Work out the finished part from the listing and answer in its coordinate system (mm). A direction names the side the tool comes from. Give positions to 0.01 mm unless a question says otherwise; leave off trailing zeros. Write each loop counter-clockwise with the first axis right and the second up, starting at its lowest first coordinate (ties: lowest second). Pieces come first, ordered by that corner, then holes.
1) Find section A-A (y = 0). Determine the outline of the cut face in (x, z), plus the area to 3 significant figures.
2) A tool of negligible diameter and unlimited length cuts with its end or side. For faces 1 (the face through (-5, 6, 12)), 2 (the face through (0, 4.8, -5.6)), 3 (the face through (0, -6, 12)), from which of +Z, -Z, +X, -X, +Y, -Y can it reach the whole face along a straight path? Write none if from no direction.
3) Straight lines are drawn through the part: probe 1 along X at (y, z) = (-4.25, -4.5); probe 2 along Y at (x, z) = (0, 3). For each, find the intervals that lie inside material, in ascending order.
4) Find section C-C (x = 0). Count the separate pieces of the cut face and the enclosed holes in it, plus the area to 3 significant figures.
5) Determine the mould class of faces 4 (the face through (0, -3, -15)), 5 (the face through (0, -4.8, -5.6)), 6 (the face through (-0.12, 4.02, -8.11)), 7 (the face through (-1.55, -5, 4)) for opening direction Z: pulls with the +Z half, pulls with the -Z half, needs draft (parallel to the pull), parting line crosses it, or undercut.
6) Given pin 1 Ø1.6 at (x, z) = (0, -9) entering from -Y; pin 2 Ø2 at (x, z) = (-5, 10.5) entering from +Y; pin 3 Ø5 at (x, z) = (-4.5, 4) entering from -Y; pin 4 Ø1.1 at (x, y) = (-2, -6.5) entering from +Z, each flat-ended and moving along its own axis, determine where each tip first touches the part or whether it passes through.
Autodesk Inventor part; units mm, degrees
ref_plane "Work Plane3" through (0, -6, 0) normal (0, 1, 0) x (-1, 0, 0)
ref_plane "YZ Plane" through (0, 0, 0) normal (1, 0, 0) x (0, 1, 0)
ref_plane "XY Plane" through (0, 0, 0) normal (0, 0, 1) x (1, 0, 0)
sketch "Sketch1" plane through (0, 0, 0) normal (0, 0, 1) x (1, 0, 0)
  line L0 (-2.1, -2.1) -> (2.1, -2.1)
  line L1 (2.1, -2.1) -> (2.1, 2.1)
  line L2 (2.1, 2.1) -> (-2.1, 2.1)
  line L3 (-2.1, 2.1) -> (-2.1, -2.1)
  line L4 (-2.1, -2.1) -> (2.1, 2.1) construction
  line L5 (2.1, -2.1) -> (-2.1, 2.1) construction
  line L6 (-6, -6) -> (6, -6)
  line L7 (6, -6) -> (6, 6)
  line L8 (6, 6) -> (-6, 6)
  line L9 (-6, 6) -> (-6, -6)
  line L10 (-6, -6) -> (6, 6) construction
  line L11 (6, -6) -> (-6, 6) construction
  line L12 (0, 6) -> (0, 2.1)
  point P0 (0, 0)
  dimension "d0" = 4.2
  dimension "d1" = 4.2
  dimension "d2" = 12
  dimension "d3" = 12
  dimension "d93" = 3.9
extrude "Extrusion1" add sketch "Sketch1" along normal mid plane 30
sketch "Sketch2" plane through (-6, 6, 15) normal (0, 1, 0) x (1, 0, 0)
  line L0 (0, 30) -> (0, 0)
  line L1 (0, 0) -> (0, 6)
  line L2 (0, 0) -> (0, 8)
  line L3 (0, 6) -> (12, 6)
  line L4 (12, 30) -> (12, 0)
  line L5 (0, 8) -> (12, 8)
  line L6 (12, 6) -> (12, 8)
  point P0 (6, 15)
  dimension "d6" = 6
  dimension "d7" = 8
  dimension "d8" = 2
extrude "Extrusion2" add sketch "Sketch2" along normal blind 2
sketch "Sketch3" plane through (-6, 6, -15) normal (0, 1, 0) x (1, 0, 0)
  line L0 (0, 0) -> (0, -30)
  line L1 (12, -30) -> (12, 0)
  line L2 (0, 0) -> (0, -22)
  line L3 (12, -30) -> (0, -30)
  line L4 (9.1, -31) -> (2.9, -31)
  line L5 (6, -6) -> (6, 0)
  circle A0 centre (6, -6) radius 1.55
  line L6 (2.8, -31) -> (4, -31)
  line L7 (9.2, -31) -> (8, -31)
  circle A1 centre (6, -6) radius 3.4
  line L8 (2.6, -6) -> (2.6, -31)
  line L9 (2.6, -6) -> (27.6, -6) construction
  line L10 (2.6, -31) -> (4, -31)
  line L11 (9.4, -6) -> (9.4, -31)
  line L12 (9.4, -6) -> (34.4, -6) construction
  line L13 (9.4, -31) -> (8, -31)
  line L14 (4.45, -6) -> (4.45, -31)
  line L15 (4.45, -6) -> (29.45, -6) construction
  line L16 (7.55, -6) -> (7.55, -31)
  line L17 (7.55, -6) -> (32.55, -6) construction
  point P0 (6, -15)
  point P1 (9.4, -30)
  point P2 (2.6, -30)
  point P3 (4.45, -30)
  point P4 (4.45, -9.0261)
  point P5 (7.55, -9.0261)
  point P6 (7.55, -30)
  dimension "d139" = 6
  dimension "d145" = 3.1
  dimension "d183" = 6.8
  dimension "d184" = 90
  dimension "d185" = 90
  dimension "d190" = 90
  dimension "d191" = 90
  dimension "d204" = 6
extrude "Extrusion3" cut sketch "Sketch3" against normal blind 2.5 contours L3 L16 A1 L11 | A1 L16 A0 L5 | L3 L8 A1 L14 | A1 L14 A0 L16 | L5 A0 L14 A1
ref_plane "Work Plane3" through (0, -6, 0) normal (0, 1, 0) x (-1, 0, 0)
sketch "Sketch16" plane through (-6, -6, -15) normal (0, -1, 0) x (1, 0, 0)
  line L0 (12, 0) -> (0, 0)
  line L1 (0, 0) -> (6, 0)
  line L2 (6, 0) -> (6, 6)
  circle A0 centre (6, 6) radius 1.55
  arc A1 (7.55, 6) -> (7.55, 6) centre (6, 6) ccw
  line L3 (10.2, 6) -> (36.7126, 6) construction
  line L4 (8.95, 32.5126) -> (7.75, 32.5126)
  line L5 (2.8, 6) -> (29.3126, 6) construction
  line L6 (7.55, 6) -> (9.4, 6)
  circle A2 centre (6, 6) radius 3.4
  line L7 (9.4, 6) -> (9.4, 32.5126)
  line L8 (9.4, 6) -> (35.9126, 6) construction
  line L9 (9.4, 32.5126) -> (7.75, 32.5126)
  line L10 (2.6, 6) -> (2.6, 32.5126)
  line L11 (2.6, 6) -> (29.1126, 6) construction
  line L12 (7.55, 6) -> (7.55, 32.5126)
  line L13 (7.55, 6) -> (34.0626, 6) construction
  line L14 (7.55, 32.5126) -> (9.4, 32.5126)
  line L15 (4.45, 6) -> (4.45, 32.5126)
  line L16 (4.45, 6) -> (30.9626, 6) construction
  line L17 (4.45, 32.5126) -> (2.6, 32.5126)
  point P0 (10.1, 6)
  point P1 (4.45, 9.0261)
  point P2 (7.55, 9.0261)
  dimension "d155" = 6
  dimension "d156" = 6
  dimension "d181" = 90
  dimension "d182" = 90
  dimension "d187" = 3.1
  dimension "d188" = 90
  dimension "d189" = 90
  dimension "d198" = 6.8
extrude "Extrusion12" cut sketch "Sketch16" against normal blind 2.5 contours A2 L15 A0 L2 | L2 A0 L6 A2 | L10 L17 L15 A2 | L6 L12 A2 | A2 L12 L14 L4 L9 L7 | L15 A2 L12 A0
sketch "Sketch17" plane through (0, -6, -9) normal (0, -1, 0) x (1, 0, 0)
  circle A0 centre (0, 0) radius 0.9
  point P0 (0, 9)
  point P1 (3.1, 0)
  dimension "d186" = 1.8
extrude "Extrusion13" cut sketch "Sketch17" against normal through all
sketch "Sketch18" plane through (0, -6, -9) normal (0, -1, 0) x (1, 0, 0)
  line L0 (0, 0) -> (0, 1)
  arc A0 (-7, 1) -> (7, 1) centre (0, 1) ccw
  line L1 (0, 1) -> (7, 1)
  line L2 (0, 1) -> (-7, 1)
  line L3 (7, 1) -> (7, -9.6793)
  line L4 (7, -9.6793) -> (-7, -9.6793)
  line L5 (-7, -9.6793) -> (-7, 1)
  point P0 (0, 9)
  dimension "d167" = 1
extrude "Extrusion14" cut sketch "Sketch18" against normal through all contours A0 L3 L4 L5
fillet "Fillet11" radius 1 2 edges at (0, 8, 7) (0, 8, 9)
fillet "Fillet12" radius 0.5 12 edges at (3.4, 3.5, 3) (-3.4, 3.5, 3) (0, 3.5, -12.4) (-1.55, 3.5, -9) (1.55, 3.5, 4.5131) (-1.55, 3.5, 4.5131) (0, -3.5, -12.4) (3.4, -3.5, 3) (-3.4, -3.5, 3) (-1.55, -3.5, -9) (1.55, -3.5, 4.5131) (-1.55, -3.5, 4.5131)
sketch "Sketch19" plane through (0, -6, -9) normal (0, -1, 0) x (1, 0, 0)
  line L0 (0, 0) -> (0, 24)
  line L1 (1.55, 24) -> (-1.55, 24)
  line L2 (3.4, 24) -> (6, 24)
  line L3 (0, 24) -> (6, 24)
  line L4 (6, 24) -> (6, 18)
  line L5 (3.4, 16) -> (6, 16)
  line L6 (-6, 16) -> (-3.4, 16)
  line L7 (6, 16) -> (-6, 16)
  line L8 (-6, 16) -> (-6, 18)
  line L9 (-6, 16) -> (-6, 18)
  line L10 (-6, 18) -> (6, 18)
  line L11 (6, 18) -> (6, 15.7444)
  point P0 (0, 9)
  point P1 (6, 16)
  point P2 (-3.4, 16)
  point P3 (3.4, 16)
  dimension "d194" = 6
extrude "Extrusion15" add sketch "Sketch19" along normal blind 2 contours L7 L6 L8 L10 L0 | L0 L10 L11 L5 L7
fillet "Fillet13" radius 1 2 edges at (0, -8, 7) (0, -8, 9)
properties part number "Nedre del av kne proto1"
Results:
1. outline: (-6, -11.61) arc R7 ccw to (-2.1, -14.68) - (-2.1, 15) - (-6, 15) - close; (2.1, -14.68) arc R7 ccw to (6, -11.61) - (6, 15) - (2.1, 15) - close
1. area: 223 mm2
2. face 1: +Z, +X, -X, +Y
2. face 2: +Y
2. face 3: +Z, +X, -X, -Y
3. probe 1: x = -6 to -3.4, -1.55 to 1.55, 3.4 to 6
3. probe 2: y = -6 to -2.1, 2.1 to 6
4. separate pieces: 4
4. enclosed holes: 0
4. area: 209 mm2
5. face 4: pulls with the -Z half
5. face 5: undercut
5. face 6: undercut
5. face 7: needs draft
6. pin 1: passes through
6. pin 2: stops at y = 6
6. pin 3: stops at y = -6
6. pin 4: stops at z = 9
